from build123d import *

# Parameters (mm, degrees)
SKETCH1_R           = 25.4
BOSS_EXTRUDE1_DEPTH = 31.75
SKETCH2_R           = 7.62
BOSS_EXTRUDE2_DEPTH = 38.1
SKETCH3_W           = 50.8
SKETCH3_H           = 76.2
BOSS_EXTRUDE3_DEPTH = 22.225
SKETCH4_R           = 6.35
CUT_EXTRUDE1_DEPTH  = 60.56828015


with BuildPart() as part:
    # Sketch1 → Boss-Extrude1 (new body)
    with BuildSketch(Plane.XY):
        Circle(SKETCH1_R)
    extrude(amount=BOSS_EXTRUDE1_DEPTH)

    # Sketch2 → Boss-Extrude2 (add)
    with BuildSketch(Plane.XY):
        with Locations(Location((0, 0, 0), (0, 0, 180))):
            Circle(SKETCH2_R)
    extrude(amount=BOSS_EXTRUDE2_DEPTH)

    # Sketch3 → Boss-Extrude3 (add)
    with BuildSketch(Plane.XY):
        Rectangle(SKETCH3_W, SKETCH3_H)
    extrude(amount=BOSS_EXTRUDE3_DEPTH)

    # Sketch4 → Cut-Extrude1 (cut, through all)
    with BuildSketch(Plane.XY):
        with Locations(Location((0, 0, 0), (0, 0, 180))):
            Circle(SKETCH4_R)
    extrude(amount=CUT_EXTRUDE1_DEPTH, mode=Mode.SUBTRACT)


solid = part.part
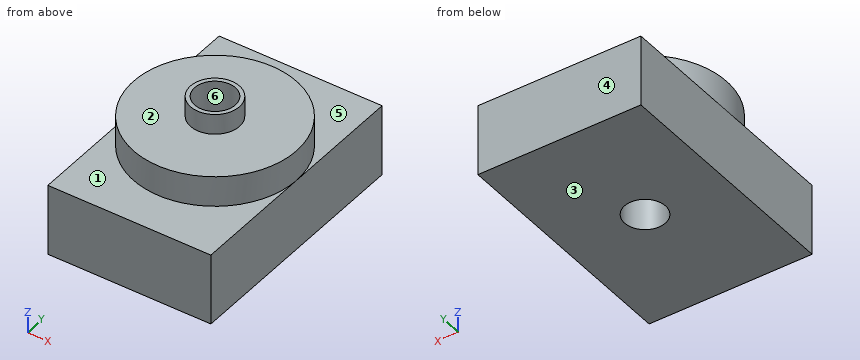
Model file for the job. Use its own axes, mm. Face numbers are marked on the shaded views. A direction names the side the tool comes from. Give positions to 0.01 mm unless a question says otherwise; leave off trailing zeros. Order: outer loops, then holes, each group sorted by start corner. A loop starts at its lowest first (then second) coordinate and runs counter-clockwise, first axis right, second up. Notation, with made-up numbers: (-39, 1) -> (-26, 1) arc R14 ccw to (-26, 18) -> close; hole circle Ø4 at (-11, 53.25). An arc over 180 degrees is marked (long way). Use CSV: the item, a comma, the result in double quotes.
1. Band-saw the part on A-A, the plane z = 19.5. Give the cut face in (x, y), then the cut area to 3 significant figures.
Outcome:
outline,"(-25.4, -38.1) -> (25.4, -38.1) -> (25.4, 38.1) -> (-25.4, 38.1) -> close; hole circle Ø12.7 at (0, 0)"
area,"3,740 mm²"
2. Drop flat-ended pins along their axis: pin 1 (3 mm diameter, centred on x = 12.5, z = 29, fed in from -Y); pin 2 (2 mm diameter, centred on x = 0.5, y = 12.5, fed in from +Z); pin 3 (6 mm diameter, centred on x = 1.5, z = 32, fed in from -Y). Give the stop position or say it passes through.
Outcome:
pin 1,"y = -22.89"
pin 2,"z = 31.75"
pin 3,"y = -25.4"
3. Band-saw the part on B-B, the plane x = 0. Give the cut face in (y, z) (3 decimals).
Outcome:
outline,"(-38.1, 0) -> (-6.35, 0) -> (-6.35, 38.1) -> (-7.62, 38.1) -> (-7.62, 31.75) -> (-25.4, 31.75) -> (-25.4, 22.225) -> (-38.1, 22.225) -> close; (6.35, 0) -> (38.1, 0) -> (38.1, 22.225) -> (25.4, 22.225) -> (25.4, 31.75) -> (7.62, 31.75) -> (7.62, 38.1) -> (6.35, 38.1) -> close"
4. Band-saw the part on C-C, the plane y = 24. Give the cut face in (x, z) (3 decimals), then the cut area to 3 significant figures.
Outcome:
outline,"(-25.4, 0) -> (25.4, 0) -> (25.4, 22.225) -> (8.316, 22.225) -> (8.316, 31.75) -> (-8.316, 31.75) -> (-8.316, 22.225) -> (-25.4, 22.225) -> close"
area,"1,290 mm²"
5. Band-saw the part on D-D, the plane x = -15.5. Give the cut face in (y, z) (3 decimals), then the cut area to 3 significant figures.
Outcome:
outline,"(-38.1, 0) -> (38.1, 0) -> (38.1, 22.225) -> (20.122, 22.225) -> (20.122, 31.75) -> (-20.122, 31.75) -> (-20.122, 22.225) -> (-38.1, 22.225) -> close"
area,"2,080 mm²"
6. Drill centre lines: line 1 along Y through (x, z) = (0, 28.5); line 2 along Y through (x, z) = (0, 16); line 3 along Z through (x, y) = (-15.5, 30) (3 decimals). Where is each one in solid material? Low to high. Write a range as from..to.
Outcome:
line 1,"-25.4..-6.35, 6.35..25.4"
line 2,"-38.1..-6.35, 6.35..38.1"
line 3,"0..22.225"
7. 3-axis set-ups, long thin cutter, end or side, ignore diameter. For the marked faces 1, 2 and 3: which of +Z, -Z, +X, -X, +Y, -Y reach the whole face in a straight line?
Outcome:
face 1,"+Z, -Y"
face 2,"+Z"
face 3,"-Z, +X, -X, +Y, -Y"
8. Mould opens along Y. For the marked faces 4, 5 and 6 say: +Y half, -Y half, draft (parallel to the pull), parting line (faces both ways), or undercut.
Outcome:
face 4,"+Y half"
face 5,"draft"
face 6,"undercut"
